```python
from build123d import *

# Parameters (mm, degrees)
EXTRUSION1_DEPTH = 18.5
ESQUISSE2_R      = 1.5
EXTRUSION2_DEPTH = 5
ESQUISSE3_R      = 4.5
ESQUISSE3_R_2    = 1.5
EXTRUSION3_DEPTH = 5
ESQUISSE4_R      = 1.5
EXTRUSION4_DEPTH = 34.008102077


with BuildPart() as part:
    # Esquisse1 → Extrusion1 (new body)
    with BuildSketch(Plane.XY):
        Polygon((-16.636265327, 18.635578947), (-16.636265327, -1.364421053), (3.363734673, -1.364421053), (3.363734673, 18.635578947), (1.863734673, 18.635578947), (1.863734673, 0.135578947), (-15.136265327, 0.135578947), (-15.136265327, 18.635578947), align=None)
    extrude(amount=EXTRUSION1_DEPTH)

    # Esquisse2 → Extrusion2 (cut)
    with BuildSketch(Plane(origin=(3.363734673, 0, 0), x_dir=(0, 0, -1), z_dir=(1, 0, 0))):
        with Locations((-14, 6.135578947)):
            Circle(ESQUISSE2_R)
    extrude(amount=-EXTRUSION2_DEPTH, mode=Mode.SUBTRACT)

    # Esquisse3 → Extrusion3 (cut)
    with BuildSketch(Plane.ZY.offset(16.636265327)):
        with Locations((8, 20.135578947)):
            Circle(ESQUISSE3_R)
        with Locations(Location((6, 4.135578947, 0), (0, 0, 270))):
            Circle(ESQUISSE3_R_2)
    extrude(amount=-EXTRUSION3_DEPTH, mode=Mode.SUBTRACT)

    # Esquisse4 → Extrusion4 (cut, through all)
    with BuildSketch(Plane.ZY.offset(16.636265327)):
        with Locations(Location((8, 10.135578947, 0), (0, 0, 270))):
            Circle(ESQUISSE4_R)
    extrude(amount=-EXTRUSION4_DEPTH, mode=Mode.SUBTRACT)


solid = part.part
```
Check sheet for the modelled part. Datum: model origin and axes. Units: mm. A direction names the side the tool comes from. Coordinates: 2 decimals unless noted, no trailing zeros. Write each loop counter-clockwise with the first axis right and the second up, starting at its lowest first coordinate (ties: lowest second). Pieces come first, ordered by that corner, then holes. Notation, with made-up numbers: (22, 15) - (52, 15) arc R27 ccw to (52, 52) - close; hole circle Ø3 at (-24.5, 63.25). An arc over 180 degrees is marked (long way). One line per question, with ' | ' between items.
Item 1: Gauge pin test, flat ends, axial feed: P1, Ø2, axis at y = 7.5, z = 13.5, coming from the +X side; P2, Ø4, axis at x = -8, y = 4, coming from the -Z side. Record the tip position at first contact, or that the pin passes through.
Determined:
P1: stops at x = 3.36 | P2: passes through
Item 2: Sectioned sample at A-A on z = 14. Record the boundary of the cut face in (x, y), plus the area to 3 significant figures.
Determined:
outline: (-16.64, -1.36) - (3.36, -1.36) - (3.36, 4.64) - (1.86, 4.64) - (1.86, 0.14) - (-15.14, 0.14) - (-15.14, 18.64) - (-16.64, 18.64) - close; (1.86, 7.64) - (3.36, 7.64) - (3.36, 18.64) - (1.86, 18.64) - close | area: 81.0 mm2
Item 3: Access from +Z, -Z, +X, -X, +Y, -Y to the whole of each face (thin tool, end or side, straight path). Record for faces 1 (the face through (2.603, 10.461, 6.536)), 2 (the face through (2.6, 6.2, 15.5)), 3 (the face through (1.864, 12, 9)), 4 (the face through (-15.897, 2.705, 6.451)), 5 (the face through (3, 18.636, 9)).
Determined:
face 1: +X, -X | face 2: +X | face 3: +Z, -Z, +Y | face 4: -X | face 5: +Z, -Z, +X, -X, +Y
Item 4: Mould release check, pull along Z, two halves, no side actions. Record for faces 6 (the face through (-6.7, -0.2, 18.5)), 7 (the face through (-15.136, 9, 11)), 8 (the face through (-15.897, 15.636, 7.922)), 9 (the face through (-6.7, -0.2, 0)): pulls with the +Z half, pulls with the -Z half, needs draft (parallel to the pull), parting line crosses it, or undercut.
Determined:
face 6: pulls with the +Z half | face 7: needs draft | face 8: undercut | face 9: pulls with the -Z half
Item 5: Sectioned sample at C-C on z = 2.75. Record the boundary of the cut face in (x, y), plus the area to 3 significant figures.
Determined:
outline: (-16.64, -1.36) - (3.36, -1.36) - (3.36, 18.64) - (1.86, 18.64) - (1.86, 0.14) - (-15.14, 0.14) - (-15.14, 18.64) - (-16.64, 18.64) - close | area: 85.5 mm2
Item 6: Thickness scan on line 1 (Y direction, x = 2.45, z = 14); line 2 (X direction, y = 14, z = 1.5); line 3 (Y direction, x = -8.5, z = 12.5). Record the ranges inside material, lowest first. Write a range as [from, to].
Determined:
line 1: y = [-1.36, 4.64], [7.64, 18.64] | line 2: x = [-16.64, -15.14], [1.86, 3.36] | line 3: y = [-1.36, 0.14]
Item 7: Sectioned sample at B-B on y = 8.25. Record the boundary of the cut face in (x, z).
Determined:
outline: (-16.64, 0) - (-15.14, 0) - (-15.14, 18.5) - (-16.64, 18.5) - close; (1.86, 0) - (3.36, 0) - (3.36, 18.5) - (1.86, 18.5) - close
Item 8: Sectioned sample at D-D on z = 8. Record the boundary of the cut face in (x, y).
Determined:
outline: (-16.64, -1.36) - (3.36, -1.36) - (3.36, 8.64) - (1.86, 8.64) - (1.86, 0.14) - (-15.14, 0.14) - (-15.14, 8.64) - (-16.64, 8.64) - close; (-16.64, 11.64) - (-15.14, 11.64) - (-15.14, 15.64) - (-16.64, 15.64) - close; (1.86, 11.64) - (3.36, 11.64) - (3.36, 18.64) - (1.86, 18.64) - close
